```python
from build123d import *

# Parameters (mm, degrees)
SKETCH_1_R          = 8
EXTRUDE_1_DEPTH     = 200
SKETCH_2_W          = 40
SKETCH_2_H          = 40
EXTRUDE_2_DEPTH     = 5
SKETCH_3_R          = 2.5
CUT_EXTRUDE_1_DEPTH = 5


with BuildPart() as part:
    # 草图1 → 凸台-拉伸1 (new body)
    with BuildSketch(Plane(origin=(0, 0, 0), x_dir=(1, 0, 0), z_dir=(0, 1, 0))):
        with Locations(Location((0, 0, 0), (0, 0, 270))):
            Circle(SKETCH_1_R)
    extrude(amount=EXTRUDE_1_DEPTH)

    # 草图2 → 凸台-拉伸2 (add)
    with BuildSketch(Plane(origin=(0, 200, 0), x_dir=(1, 0, 0), z_dir=(0, 1, 0))):
        Rectangle(SKETCH_2_W, SKETCH_2_H)
    extrude(amount=EXTRUDE_2_DEPTH)

    # 草图3 → 切除-拉伸1 (cut)
    with BuildSketch(Plane(origin=(0, 205, 0), x_dir=(1, 0, 0), z_dir=(0, 1, 0))):
        with Locations(Location((-15, 15, 0), (0, 0, 270))):
            Circle(SKETCH_3_R)
        with Locations(Location((15, 15, 0), (0, 0, 270))):
            Circle(SKETCH_3_R)
        with Locations(Location((15, -15, 0), (0, 0, 270))):
            Circle(SKETCH_3_R)
        with Locations(Location((-15, -15, 0), (0, 0, 270))):
            Circle(SKETCH_3_R)
    extrude(amount=-CUT_EXTRUDE_1_DEPTH, mode=Mode.SUBTRACT)


solid = part.part
```
Geometry: final body of the model. Coordinates: model frame, mm. A direction names the side the tool comes from. Coordinates: 2 decimals unless noted, no trailing zeros. Order: outer loops, then holes, each group sorted by start corner. A loop starts at its lowest first (then second) coordinate and runs counter-clockwise, first axis right, second up. Notation, with made-up numbers: (71, -28.75) - (92, -28.75) arc R21 cw to (92, -16.75) - close; hole circle Ø5 at (52, 79.5). An arc over 180 degrees is marked (long way). Write each question's results on one line, items separated by ' | '.
1) Pin query (flat end, axial travel): pin 1 (3 mm diameter, centred on x = 8, y = 170, fed in from +Z); pin 2 (5 mm diameter, centred on x = -1, y = 67, fed in from -Z); pin 3 (12 mm diameter, centred on y = 93, z = -1.5, fed in from -X). Return the tip coordinate at first contact, or that it passes through.
Results list:
pin 1: z = 4.66 | pin 2: z = -8 | pin 3: x = -8
2) Pull-direction query (Z, two-part tool) for faces 1 (the cylindrical face through (-16.5, 202.5, -17)), 2 (the cylindrical face through (-7.81, 98.6, -1.73)), 3 (the flat face through (0, 202, 20)); classes: pulls with the +Z half, pulls with the -Z half, needs draft (parallel to the pull), parting line crosses it, or undercut.
Results list:
face 1: undercut | face 2: parting line crosses it | face 3: pulls with the +Z half
3) Section C-C, the plane z = 0. Return loops of the section in (x, y).
Results list:
outline: (-20, 200) - (-8, 200) - (-8, 0) - (8, 0) - (8, 200) - (20, 200) - (20, 205) - (-20, 205) - close
4) Line query: line 1 (X direction, y = 201.8, z = -15); line 2 (X direction, y = 68, z = -0.5); line 3 (Y direction, x = -1, z = 11). Output: solid intervals per line, ascending. Write a range as from..to.
Results list:
line 1: -20..-17.5, -12.5..12.5, 17.5..20 | line 2: -7.98..7.98 | line 3: 200..205
5) Section D-D, the plane y = 156. Return loops of the section in (x, z).
Results list:
outline: circle Ø16 at (0, 0)
6) Section B-B, the plane z = 15.5. Return loops of the section in (x, y).
Results list:
outline: (-20, 200) - (-17.45, 200) - (-17.45, 205) - (-20, 205) - close; (-12.55, 200) - (12.55, 200) - (12.55, 205) - (-12.55, 205) - close; (17.45, 200) - (20, 200) - (20, 205) - (17.45, 205) - close
7) Section A-A, the plane x = 15. Return loops of the section in (y, z), plus the area to 3 significant figures.
Results list:
outline: (200, -20) - (205, -20) - (205, -17.5) - (200, -17.5) - close; (200, -12.5) - (205, -12.5) - (205, 12.5) - (200, 12.5) - close; (200, 17.5) - (205, 17.5) - (205, 20) - (200, 20) - close | area: 150 mm^2
8) Set-up query: faces 4 (the flat face through (9, 200, 0)), 5 (the flat face through (-20, 202, 0)). Return all of +Z, -Z, +X, -X, +Y, -Y with unobstructed straight access to the full face (end or side cutting, diameter ignored); none if empty.
Results list:
face 4: -Y | face 5: +Z, -Z, -X, +Y, -Y
